```python
from build123d import *

# Parameters (mm, degrees)
SKETCH1_W      = 21
SKETCH1_H      = 4
SKETCH2_R      = 1.5
EXTRUDE4_DEPTH = 26.632011236
SKETCH3_R      = 1.5
EXTRUDE5_DEPTH = 10


with BuildPart() as part:
    # Sketch1 → Revolve1 (revolve)
    with BuildSketch(Plane.XY, mode=Mode.PRIVATE) as revolve1_sk:
        with Locations((10.5, 2)):
            Rectangle(SKETCH1_W, SKETCH1_H)
        Polygon((21, 4), (21, 0), (25, 0), (25, 2.75), align=None)
    revolve(revolve1_sk.sketch.rotate(Axis((25, 0, 0), (-1, 0, 0)), 90), axis=Axis((25, 0, 0), (-1, 0, 0)))

    # Sketch2 → Extrude4 (cut, through all)
    with BuildSketch(Plane(origin=(0, 0, 0), x_dir=(0, 0, -1), z_dir=(1, 0, 0))):
        Circle(SKETCH2_R)
    extrude(amount=EXTRUDE4_DEPTH, mode=Mode.SUBTRACT)

    # Sketch3 → Extrude5 (cut)
    with BuildSketch(Plane(origin=(0, 0, 0), x_dir=(1, 0, 0), z_dir=(0, 1, 0))):
        with Locations(Location((4, 0, 0), (0, 0, 90))):
            Circle(SKETCH3_R)
    extrude(amount=EXTRUDE5_DEPTH, mode=Mode.SUBTRACT)


solid = part.part
```
The listing builds one solid part. Answer for the finished solid, in the listing's coordinates (mm). Coordinates: 2 decimals unless noted, no trailing zeros. Write each loop counter-clockwise with the first axis right and the second up, starting at its lowest first coordinate (ties: lowest second). Pieces come first, ordered by that corner, then holes. Notation, with made-up numbers: M 63.25,75.5 L 73.25,75.5 A19 ccw 73.25,85.5 Z; hole C 89,8 d11. An arc over 180 degrees is marked long. Use a Markdown table: item, result. Add a question column.
1. Given P1, Ø1.5, axis at x = 21.5, y = 1, coming from the +Z side; P2, Ø1.5, axis at x = 13, z = -1.5, coming from the +Y side; P3, Ø1, axis at x = 12, z = 2.5, coming from the +Y side, each flat-ended and moving along its own axis, determine where each tip first touches the part or whether it passes through.
2. Section D-D (x = 21.25) is taken. Give the vertices of the cut face in (y, z).
3. Section B-B (x = 13.5) is taken. Give the vertices of the cut face in (y, z).
4. Section C-C (x = 4) is taken. Give the vertices of the cut face in (y, z), plus the area to 3 significant figures.
5. Straight lines are drawn through the part: line 1 along X through (y, z) = (1.6, 0); line 2 along Z through (x, y) = (4, 1.45); line 3 along Y through (x, z) = (10.5, -1.25). For each, find the intervals that lie inside material, in ascending order. Write a range as [from, to].
6. Section A-A (z = 0) is taken. Give the vertices of the cut face in (x, y), plus the area to 4 significant figures.
7. For a pull along Z with two mould halves and no side action, classify faces 1 (the flat face through (0, 0, 2)), 2 (the cylindrical face through (12.325, -1.464, 0.325)), 3 (the conical face through (23.861, -0.933, -2.963)), 4 (the cylindrical face through (4.9, 2.4, 1.2)) as +Z half, -Z half, draft (parallel to the pull), parting line (faces both ways), or undercut.
Data:
| question | item | result |
|---|---|---|
| 1 | P1 | stops at z = 3.98 |
| 1 | P2 | stops at y = 3.93 |
| 1 | P3 | stops at y = 3.46 |
| 2 | outline | C 0,0 d7.84; hole C 0,0 d3 |
| 3 | outline | C 0,0 d8; hole C 0,0 d3 |
| 4 | outline | M 0,-1.5 A1.5 cw 0,1.5 L 3.71,1.5 A4 ccw long 3.71,-1.5 Z |
| 4 | area | 35.0 mm2 |
| 5 | line 1 | x = [0, 2.5], [5.5, 25] |
| 5 | line 2 | z = [-3.73, -1.5], [1.5, 3.73] |
| 5 | line 3 | y = [-3.8, -0.83], [0.83, 3.8] |
| 6 | outline | M 0,-4 L 21,-4 L 25,-2.75 L 25,-1.5 L 0,-1.5 Z; M 0,1.5 L 2.5,1.5 L 2.5,4 L 0,4 Z; M 5.5,1.5 L 25,1.5 L 25,2.75 L 21,4 L 5.5,4 Z |
| 6 | area | 112.5 mm2 |
| 7 | face 1 | draft |
| 7 | face 2 | undercut |
| 7 | face 3 | parting line |
| 7 | face 4 | undercut |
